Could you check a few things on this model? Use its own coordinates, in mm. Coordinates: 2 decimals unless noted, no trailing zeros. Order: outer loops, then holes, each group sorted by start corner. A loop starts at its lowest first (then second) coordinate and runs counter-clockwise, first axis right, second up. Notation, with made-up numbers: (-2, 79) - (30, 79) arc R22 cw to (30, 100) - close; hole circle Ø4 at (80, 43.5). An arc over 180 degrees is marked (long way). Answer as CSV lines item,"result". Start each with the question number.
1. For pin 1 (8 mm diameter, centred on y = 76.5, z = 259, fed in from -X); pin 2 (1.5 mm diameter, centred on y = 86.5, z = 262.5, fed in from -X); pin 3 (1 mm diameter, centred on y = 79.5, z = 256, fed in from +X), each with a flat end and sliding along its axis, tell me the tip position at first contact or that it passes through.
2. I need wall thicknesses on probe 1 along Y at (x, z) = (0, 265.25); probe 2 along Y at (x, z) = (-2, 256.25); probe 3 along X at (y, z) = (82, 258). Which ranges of each line are inside material? Lowest first, please.
3. I want a section at C-C, the plane z = 256.75. List the corners of the cut face in (x, y) for me.
4. I want a section at B-B, the plane y = 83. List the corners of the cut face in (x, z) for me.
5. I want a section at D-D, the plane x = 4.5. List the corners of the cut face in (y, z) for me.
6. I want a section at A-A, the plane x = 0. List the corners of the cut face in (y, z) for me.
from build123d import *

# Parameters (mm, degrees)
CYLINDER670_R     = 2.65
CYLINDER670_DEPTH = 40
CYLINDER669_R     = 8
CYLINDER669_DEPTH = 17


with BuildPart() as obj1:
    # Cylinder670 → Cylinder670 (new body)
    with BuildSketch(Plane(origin=(0, 83, 232), x_dir=(1, 0, 0), z_dir=(0, 0, 1))):
        Circle(CYLINDER670_R)
    extrude(amount=CYLINDER670_DEPTH)


with BuildPart() as cut268:
    # Cylinder669 → Cylinder669 (new body)
    with BuildSketch(Plane(origin=(0, 83, 252), x_dir=(1, 0, 0), z_dir=(0, 0, 1))):
        Circle(CYLINDER669_R)
    extrude(amount=CYLINDER669_DEPTH)

    # Cut268: cut obj1
    add(obj1.part, mode=Mode.SUBTRACT)


solid = cut268.part
Solved:
1,pin 1,"stops at x = -7.6"
1,pin 2,"stops at x = -7.51"
1,pin 3,"stops at x = 7.42"
2,probe 1,"y = 75 to 80.35, 85.65 to 91"
2,probe 2,"y = 75.25 to 81.26, 84.74 to 90.75"
2,probe 3,"x = -7.94 to -2.45, 2.45 to 7.94"
3,outline,"circle Ø16 at (0, 83); hole circle Ø5.3 at (0, 83)"
4,outline,"(-8, 252) - (-2.65, 252) - (-2.65, 269) - (-8, 269) - close; (2.65, 252) - (8, 252) - (8, 269) - (2.65, 269) - close"
5,outline,"(76.39, 252) - (89.61, 252) - (89.61, 269) - (76.39, 269) - close"
6,outline,"(75, 252) - (80.35, 252) - (80.35, 269) - (75, 269) - close; (85.65, 252) - (91, 252) - (91, 269) - (85.65, 269) - close"
